Can you work these out from the drawing? Everything is in mm from the part's minimum corner. Round coordinates to 2 decimals unless told otherwise and drop trailing zeros. Loops run counter-clockwise (first coordinate to the right, second up) from the corner with the lowest first, then second, coordinate; pieces in that order, holes last. Notation, with made-up numbers: M 86,35 L 110,35 A21 cw 110,48 Z; hole C 82,-32.75 d4. An arc over 180 degrees is marked long. Use a Markdown table: item, result.
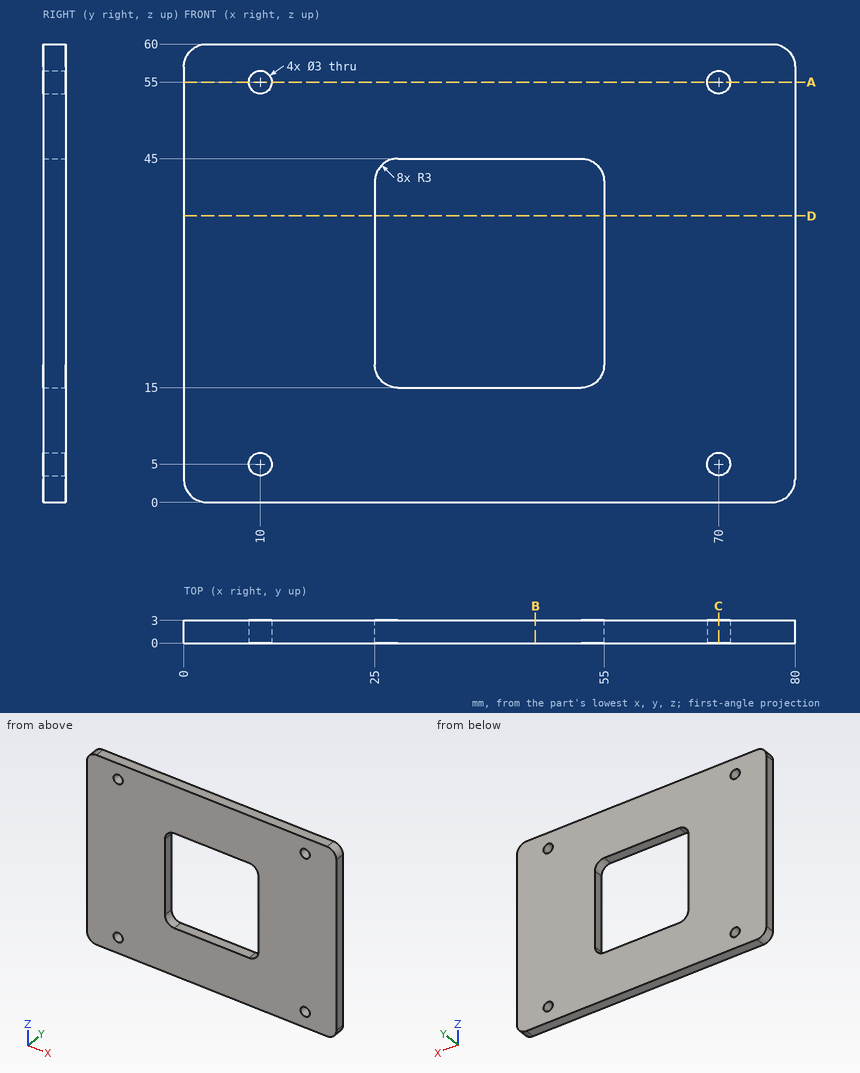
Q1. Imagine slicing it at B-B, the plane x = 46. Please give me the cut outline in (y, z), then the cut area to 3 significant figures.
Return value:
| item | result |
|---|---|
| outline | M 0,0 L 3,0 L 3,15 L 0,15 Z; M 0,45 L 3,45 L 3,60 L 0,60 Z |
| area | 90.0 mm^2 |
Q2. Imagine slicing it at A-A, the plane z = 55. Please give me the cut outline in (x, y), then the cut area to 3 significant figures.
Return value:
| item | result |
|---|---|
| outline | M 0,0 L 8.5,0 L 8.5,3 L 0,3 Z; M 11.5,0 L 68.5,0 L 68.5,3 L 11.5,3 Z; M 71.5,0 L 80,0 L 80,3 L 71.5,3 Z |
| area | 222 mm^2 |
Q3. Imagine slicing it at D-D, the plane z = 37.5. Please give me the cut outline in (x, y), then the cut area to 3 significant figures.
Return value:
| item | result |
|---|---|
| outline | M 0,0 L 25,0 L 25,3 L 0,3 Z; M 55,0 L 80,0 L 80,3 L 55,3 Z |
| area | 150 mm^2 |
Q4. I need wall thicknesses on line 1 (Z direction, x = 70, y = 1.85); line 2 (X direction, y = 0.95, z = 5); line 3 (X direction, y = 1.65, z = 18). Which ranges of each line are inside material? Lowest first, please. Write a range as from..to.
Return value:
| item | result |
|---|---|
| line 1 | z = 0..3.5, 6.5..53.5, 56.5..60 |
| line 2 | x = 0..8.5, 11.5..68.5, 71.5..80 |
| line 3 | x = 0..25, 55..80 |
Q5. Imagine slicing it at C-C, the plane x = 70. Please give me the cut outline in (y, z).
Return value:
| item | result |
|---|---|
| outline | M 0,0 L 3,0 L 3,3.5 L 0,3.5 Z; M 0,6.5 L 3,6.5 L 3,53.5 L 0,53.5 Z; M 0,56.5 L 3,56.5 L 3,60 L 0,60 Z |
